Here's how the part is built. I have some questions about the finished solid (model axes, mm). A direction names the side the tool comes from. Give positions to 0.01 mm unless a question says otherwise; leave off trailing zeros. Loops run counter-clockwise (first coordinate to the right, second up) from the corner with the lowest first, then second, coordinate; pieces in that order, holes last. Notation, with made-up numbers: (-26, 44.25) - (-6, 44.25) arc R24 cw to (-6, 61.25) - close; hole circle Ø7 at (8.5, 23). An arc over 180 degrees is marked (long way). Return JSON: item names as keys, results as strings. Group by question number.
(1) For P1, Ø4, axis at x = -13.5, y = 34, coming from the +Z side; P2, Ø0.8, axis at x = -1, y = 1.5, coming from the +Z side; P3, Ø10, axis at y = 62, z = 13, coming from the -X side, each with a flat end and sliding along its axis, tell me the tip position at first contact or that it passes through.
(2) If we section it at D-D (z = -9): Please give me the cut outline in (x, y) (1 decimal), then the cut area to 3 significant figures.
(3) If we mould it in two halves opening along Y, with no side actions, what happens to faces 1 (the flat face through (1, 0, -8)), 2 (the flat face through (0, 2.5, -12)), 3 (the flat face through (-2.819, 1, -15)), 4 (the flat face through (-16.4, 15, 1))? For each: released by +Y, released by -Y, zero draft, split by the parting line, or undercut.
(4) If we section it at A-A (z = 9.5): Please give me the cut outline in (x, y) (1 decimal).
(5) I need wall thicknesses on probe 1 along Y at (x, z) = (12.5, 1) (3 decimals); probe 2 along Z at (x, y) = (0, 16); probe 3 along Y at (x, z) = (9.5, 0.5) (3 decimals). Which ranges of each line are inside material? Lowest first, please. Write a range as [from, to].
(6) On a 3-axis mill with a long thin cutter (end or side, diameter ignored), from which of +Z, -Z, +X, -X, +Y, -Y can I reach the whole of each face in a straight line? I mean faces 5 (the flat face through (-2, 2.5, 14)), 6 (the flat face through (-1, 1, -17.513)), 7 (the flat face through (-1, 1, 17.513)), 8 (the flat face through (8.53, 75.82, 8.61)), 9 (the flat face through (-2.819, 1, 16)). Say none if no direction works.
(7) If we section it at B-B (x = -11): Please give me the cut outline in (y, z) (3 decimals).
(8) If we section it at C-C (y = 12): Please give me the cut outline in (x, z) (1 decimal).
```python
from build123d import *

# Parameters (mm, degrees)
BOSS_EXTRUDE1_DEPTH = 2.5
CUT_EXTRUDE1_REACH  = 26.645
SKETCH2_R           = 1.715
SKETCH2_R_2         = 8.98
SKETCH3_R           = 2.6543
BOSS_EXTRUDE2_DEPTH = 70.305
BOSS_EXTRUDE3_START = 4
SKETCH4_R           = 21
SKETCH4_R_2         = 8.98
BOSS_EXTRUDE3_DEPTH = 4
SKETCH6_R           = 21
SKETCH6_R_2         = 8.98
BOSS_EXTRUDE4_DEPTH = 2
CUT_EXTRUDE3_START  = -15
SKETCH7_R           = 1.715
CUT_EXTRUDE3_DEPTH  = 15
SKETCH8_R           = 8.98
CUT_EXTRUDE4_DEPTH  = 2
BOSS_EXTRUDE6_REACH = 82.451
SKETCH10_R          = 12.48
SKETCH10_R_2        = 8.98
SKETCH12_R          = 21
SKETCH12_R_2        = 12.48
CUT_EXTRUDE5_DEPTH  = 57.805


with BuildPart() as part:
    # Sketch1 → Boss-Extrude1 (new body)
    with BuildSketch(Plane(origin=(0, 0, 0), x_dir=(1, 0, 0), z_dir=(0, 1, 0))):
        with BuildLine():
            Line((0.597960958, 12.236443242), (0.597960958, 17.5133))
            Line((0.597960958, 17.5133), (-2.819411684, 17.5133))
            Line((-2.819411684, 17.5133), (-2.819411684, 11.976881697))
            ThreePointArc((-2.819411684, 11.976881697), (-9.752212861, 8.278991937), (-13.533031252, 1.391065316))
            ThreePointArc((-13.533031252, 1.391065316), (-17.156497956, -0.999626805), (-13.683409812, -3.603965207))
            ThreePointArc((-13.683409812, -3.603965207), (-10.042516815, -11.01106651), (-2.819411684, -15.004561697))
            Line((-2.819411684, -15.004561697), (-2.819411684, -17.5133))
            Line((-2.819411684, -17.5133), (0.597960958, -17.5133))
            Line((0.597960958, -17.5133), (0.597960958, -15.264123242))
            ThreePointArc((0.597960958, -15.264123242), (9.161591247, -11.721092084), (13.538839655, -3.55233882))
            ThreePointArc((13.538839655, -3.55233882), (17.156522938, -1.000460972), (13.393344487, 1.331534062))
            ThreePointArc((13.393344487, 1.331534062), (8.853545908, 8.96396608), (0.597960958, 12.236443242))
        make_face()
    extrude(amount=BOSS_EXTRUDE1_DEPTH)

    # Sketch2 → Cut-Extrude1 (cut, up to next)
    with BuildSketch(Plane(origin=(0, 2.5, 0), x_dir=(1, 0, 0), z_dir=(0, 1, 0)), mode=Mode.PRIVATE) as cut_extrude1_sk1:
        with Locations(Location((-14.5034, -1.0795, 0), (0, 0, 270))):
            Circle(SKETCH2_R)
    cut_extrude1_tool1 = extrude(cut_extrude1_sk1.sketch, amount=-CUT_EXTRUDE1_REACH, mode=Mode.PRIVATE) & part.part
    # Sketch2 → Cut-Extrude1 (cut, up to next)
    with BuildSketch(Plane(origin=(0, 2.5, 0), x_dir=(1, 0, 0), z_dir=(0, 1, 0)), mode=Mode.PRIVATE) as cut_extrude1_sk2:
        with Locations(Location((14.5034, -1.0795, 0), (0, 0, 270))):
            Circle(SKETCH2_R)
    cut_extrude1_tool2 = extrude(cut_extrude1_sk2.sketch, amount=-CUT_EXTRUDE1_REACH, mode=Mode.PRIVATE) & part.part
    # Sketch2 → Cut-Extrude1 (cut, up to next)
    with BuildSketch(Plane(origin=(0, 2.5, 0), x_dir=(1, 0, 0), z_dir=(0, 1, 0)), mode=Mode.PRIVATE) as cut_extrude1_sk3:
        with Locations(Location((-0.0762, -1.51384, 0), (0, 0, 270))):
            Circle(SKETCH2_R_2)
    cut_extrude1_tool3 = extrude(cut_extrude1_sk3.sketch, amount=-CUT_EXTRUDE1_REACH, mode=Mode.PRIVATE) & part.part
    add(cut_extrude1_tool1.solids().sort_by_distance((-14.5034, 2.5, 1.0795))[0], mode=Mode.SUBTRACT)
    add(cut_extrude1_tool2.solids().sort_by_distance((14.5034, 2.5, 1.0795))[0], mode=Mode.SUBTRACT)
    add(cut_extrude1_tool3.solids().sort_by_distance((-0.0762, 2.5, 1.51384))[0], mode=Mode.SUBTRACT)

    # Sketch3 → Boss-Extrude2 (add)
    with BuildSketch(Plane(origin=(0, 2.5, 0), x_dir=(1, 0, 0), z_dir=(0, 1, 0))):
        with Locations(Location((-14.5034, -1.0795, 0), (0, 0, 68.556492541))):
            Circle(SKETCH3_R)
        with Locations(Location((14.5034, -1.0795, 0), (0, 0, 114.72164566))):
            Circle(SKETCH3_R)
    extrude(amount=BOSS_EXTRUDE2_DEPTH)

    # Sketch4 → Boss-Extrude3 (add)
    with BuildSketch(Plane(origin=(0, 72.805, 0), x_dir=(1, 0, 0), z_dir=(0, 1, 0)).offset(BOSS_EXTRUDE3_START)):
        with Locations(Location((-0.0762, -1.51384, 0), (0, 0, 270))):
            Circle(SKETCH4_R)
        with Locations(Location((-0.0762, -1.51384, 0), (0, 0, 270))):
            Circle(SKETCH4_R_2, mode=Mode.SUBTRACT)
    extrude(amount=-BOSS_EXTRUDE3_DEPTH)

    # Sketch6 → Boss-Extrude4 (add)
    with BuildSketch(Plane(origin=(0, 37.805, 0), x_dir=(-1, 0, 0), z_dir=(0, -1, 0))):
        with Locations(Location((0.0762, -1.51384, 0), (0, 0, 90))):
            Circle(SKETCH6_R)
        with Locations(Location((0.0762, -1.51384, 0), (0, 0, 270))):
            Circle(SKETCH6_R_2, mode=Mode.SUBTRACT)
    extrude(amount=BOSS_EXTRUDE4_DEPTH)

    # Sketch7 → Cut-Extrude3 (cut)
    with BuildSketch(Plane.XZ.offset(CUT_EXTRUDE3_START)):
        with Locations(Location((-14.5034, 1.0795, 0), (0, 0, 90))):
            Circle(SKETCH7_R)
        with Locations(Location((14.5034, 1.0795, 0), (0, 0, 90))):
            Circle(SKETCH7_R)
    extrude(amount=CUT_EXTRUDE3_DEPTH, mode=Mode.SUBTRACT)

    # Sketch8 → Cut-Extrude4 (cut)
    with BuildSketch(Plane(origin=(0, 76.805, 0), x_dir=(1, 0, 0), z_dir=(0, 1, 0))):
        with BuildLine():
            Line((-10.0762, -1.51384), (-7.3262, -15.51384))
            ThreePointArc((-7.3262, -15.51384), (-0.0762, -17.51384), (7.1738, -15.51384))
            Line((7.1738, -15.51384), (9.9238, -1.51384))
            Line((9.9238, -1.51384), (7.1738, 12.48616))
            ThreePointArc((7.1738, 12.48616), (-0.0762, 14.48616), (-7.3262, 12.48616))
            Line((-7.3262, 12.48616), (-10.0762, -1.51384))
        make_face()
        with Locations(Location((-0.0762, -1.51384, 0), (0, 0, 270))):
            Circle(SKETCH8_R, mode=Mode.SUBTRACT)
    extrude(amount=-CUT_EXTRUDE4_DEPTH, mode=Mode.SUBTRACT)

    # Boss-Extrude6: up to this face of the body (flat: up to its plane)
    boss_extrude6_end = Plane(part.part.faces().sort_by_distance((-0.0762, 72.805, -18.892190304))[0])
    # Sketch10 → Boss-Extrude6 (add, up to the picked face)
    with BuildSketch(Plane(origin=(0, 2.5, 0), x_dir=(1, 0, 0), z_dir=(0, 1, 0)), mode=Mode.PRIVATE) as boss_extrude6_sk1:
        with Locations((-0.0762, -1.51384)):
            Circle(SKETCH10_R)
        with Locations(Location((-0.0762, -1.51384, 0), (0, 0, 270))):
            Circle(SKETCH10_R_2, mode=Mode.SUBTRACT)
    boss_extrude6_tool1 = split(extrude(boss_extrude6_sk1.sketch, amount=BOSS_EXTRUDE6_REACH, mode=Mode.PRIVATE), bisect_by=boss_extrude6_end, keep=Keep.BOTH, mode=Mode.PRIVATE)
    add(boss_extrude6_tool1.solids().sort_by(Axis((-12.203212, 2.5, 1.51384), (0, 1, 0)))[0])

    # Sketch12 → Cut-Extrude5 (cut)
    with BuildSketch(Plane.XZ.offset(-15)):
        with Locations(Location((-0.0762, 1.51384, 0), (0, 0, 90))):
            Circle(SKETCH12_R)
        with Locations(Location((-0.0762, 1.51384, 0), (0, 0, 189.400360909))):
            Circle(SKETCH12_R_2, mode=Mode.SUBTRACT)
    extrude(amount=-CUT_EXTRUDE5_DEPTH, mode=Mode.SUBTRACT)


solid = part.part
```
Values:
{
 "1": {"P1": "z = 6.54", "P2": "z = 17.51", "P3": "x = -10.74"},
 "2": {"outline": "(-18.3, 72.8) - (-6.8, 72.8) - (-6.8, 2.5) - (-9, 2.5) - (-9, 0) - (8.8, 0) - (8.8, 2.5) - (6.6, 2.5) - (6.6, 72.8) - (18.1, 72.8) - (18.1, 76.8) - (7.9, 76.8) - (7.9, 74.8) - (-8, 74.8) - (-8, 76.8) - (-18.3, 76.8) - close", "area": "1,100 mm2"},
 "3": {"face 1": "released by -Y", "face 2": "undercut", "face 3": "zero draft", "face 4": "undercut"},
 "4": {"outline": "(-19.5, 72.8) - (-9.7, 72.8) - (-9.7, 2.5) - (-11.3, 2.5) - (-11.3, 0) - (-4.2, 0) - (-4.2, 74.8) - (-8.5, 74.8) - (-8.5, 76.8) - (-19.5, 76.8) - close; (4, 0) - (11.1, 0) - (11.1, 2.5) - (9.5, 2.5) - (9.5, 72.8) - (19.3, 72.8) - (19.3, 76.8) - (8.4, 76.8) - (8.4, 74.8) - (4, 74.8) - close"},
 "5": {"probe 1": "[0, 15], [72.805, 76.805]", "probe 2": "[-10.97, -7.47], [10.49, 13.99]", "probe 3": "[0, 74.805]"},
 "6": {"face 5": "+Z", "face 6": "-Z, +X, -X, -Y", "face 7": "+Z, +X, -X, -Y", "face 8": "+Y", "face 9": "+Z, -X, -Y"},
 "7": {"outline": "(0, -6.864) - (2.5, -6.864) - (2.5, -4.521) - (72.805, -4.521) - (72.805, -16.421) - (76.805, -16.421) - (76.805, 19.449) - (72.805, 19.449) - (72.805, 7.549) - (2.5, 7.549) - (2.5, 9.892) - (0, 9.892) - close"},
 "8": {"outline": "(-12.5, 2.8) arc R2.7 ccw (long way) to (-12.4, -0.5) arc R12.5 ccw to (12.3, -0.3) arc R2.7 ccw (long way) to (12.4, 2.6) arc R12.5 ccw to start; hole circle Ø3.4 at (-14.5, 1.1); hole circle Ø18 at (-0.1, 1.5); hole circle Ø3.4 at (14.5, 1.1)"}
}
